Geometry: final body of the model. Coordinates: model frame, mm. Face numbers are marked on the shaded views. A direction names the side the tool comes from. Give positions to 0.01 mm unless a question says otherwise; leave off trailing zeros. Order: outer loops, then holes, each group sorted by start corner. A loop starts at its lowest first (then second) coordinate and runs counter-clockwise, first axis right, second up. Notation, with made-up numbers: M 25,-21.75 L 62,-21.75 A32 ccw 62,14.25 Z; hole C -34.5,0.25 d2. An arc over 180 degrees is marked long. Use CSV: the item, a comma, the result in double quotes.
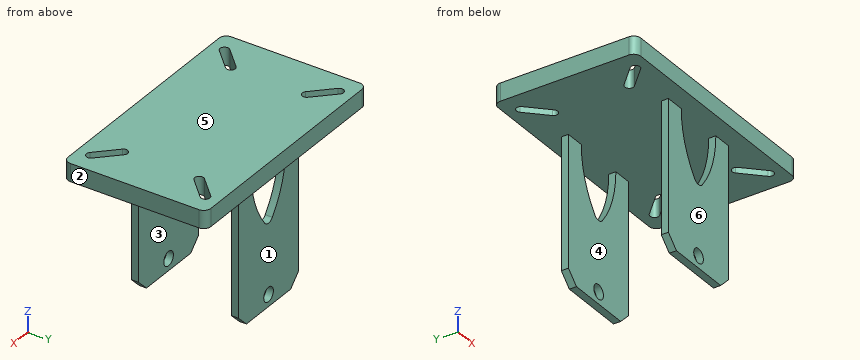
Autodesk Inventor part; units mm, degrees
ref_plane "Arbeitsebene1" through (0, 6, 0) normal (0, 1, 0) x (-1, 0, 0)
ref_plane "Arbeitsebene2" through (0, 6, 0) normal (0, 1, 0) x (-1, 0, 0)
ref_plane "YZ Plane" through (0, 0, 0) normal (1, 0, 0) x (0, 1, 0)
sketch "Skizze1" plane through (0, 0, 0) normal (0, 0, 1) x (1, 0, 0)
  line L0 (0, 0) -> (20, 0)
  line L1 (20, 0) -> (20, 12)
  line L2 (20, 12) -> (0, 12)
  line L3 (0, 12) -> (0, 0)
  point P0 (0, 6)
  dimension "d0" = 20
  dimension "d1" = 12
extrude "Extrusion1" add sketch "Skizze1" along normal blind 1.5
sketch "Skizze2" plane through (0, 0, 1.5) normal (0, 0, 1) x (1, 0, 0)
  line L0 (1.6868, 10.8132) -> (3.3132, 9.1868) construction
  line L1 (1.4217, 10.548) -> (3.048, 8.9217)
  line L2 (3.5783, 9.452) -> (1.952, 11.0783)
  arc A0 (1.952, 11.0783) -> (1.4217, 10.548) centre (1.6868, 10.8132) ccw
  arc A1 (3.048, 8.9217) -> (3.5783, 9.452) centre (3.3132, 9.1868) ccw
  line L3 (0, 12) -> (0, 0)
  line L4 (18.3132, 10.8132) -> (16.6868, 9.1868) construction
  line L5 (18.5783, 10.548) -> (16.952, 8.9217)
  line L6 (16.4217, 9.452) -> (18.048, 11.0783)
  arc A2 (18.5783, 10.548) -> (18.048, 11.0783) centre (18.3132, 10.8132) ccw
  arc A3 (16.4217, 9.452) -> (16.952, 8.9217) centre (16.6868, 9.1868) ccw
  line L7 (20, 0) -> (20, 12)
  line L8 (0, 0) -> (20, 0)
  line L9 (10, 0) -> (10, 12) construction
  line L10 (20, 12) -> (0, 12)
  point P0 (2.5, 10)
  point P1 (17.5, 10)
  dimension "d7" = 15
  dimension "d8" = 7.5
  dimension "d9" = 0.75
  dimension "d10" = 2
  dimension "d11" = 2.3
  dimension "d12" = 45
extrude "Extrusion2" cut sketch "Skizze2" against normal up to surface (1.5 mm away) contours A0 L2 A1 L1 | L5 A3 L6 A2
ref_plane "Arbeitsebene1" through (0, 6, 0) normal (0, 1, 0) x (-1, 0, 0)
mirror "Spiegeln1" about plane through (0, 6, 0) normal (0, 1, 0) of "Extrusion2"
sketch "Skizze3" plane through (0, 0, 0) normal (0, 0, -1) x (-1, 0, 0)
  line L0 (-20, 12) -> (0, 12)
  line L1 (-10, 12) -> (-10, 0) construction
  line L2 (0, 0) -> (-20, 0)
  line L3 (-6.25, 10.5) -> (-13.75, 10.5)
  line L4 (-13.75, 10.5) -> (-13.75, 9.9)
  line L5 (-13.75, 9.9) -> (-6.25, 9.9)
  line L6 (-6.25, 9.9) -> (-6.25, 10.5)
  dimension "d16" = 1.5
  dimension "d17" = 7.5
  dimension "d18" = 0.6
extrude "Extrusion3" add sketch "Skizze3" along normal blind 12
chamfer "Fasen1" distance 1 angle 45 2 edges at (13.75, 10.2, -12) (6.25, 10.2, -12)
sketch "Skizze4" plane through (6.25, 10.5, 0) normal (0, 1, 0) x (1, 0, 0)
  line L0 (7.5, 0) -> (0, 0)
  line L1 (3.75, 0) -> (3.75, 5.4569) construction
  arc A0 (5.9, 0) -> (3.75, 5.4569) centre (-2.1, 0) ccw
  arc A1 (3.75, 5.4569) -> (1.6, 0) centre (9.6, 0) ccw
  line L2 (13.75, 0) -> (-6.25, 0)
  line L3 (7.5, 0) -> (7.5, 11)
  dimension "d24" = 8
  dimension "d25" = 1.6
extrude "Extrusion4" cut sketch "Skizze4" against normal up to surface (0.6 mm away)
fillet "Rundung1" radius 0.6 1 edges at (10, 10.2, -5.4569)
sketch "Skizze5" plane through (7.25, 10.5, -12) normal (0, 1, 0) x (1, 0, 0)
  circle A0 centre (2.75, -1) radius 0.6
  line L0 (0, 0) -> (5.5, 0)
  line L1 (-1, -12) -> (-1, -1)
  point P0 (-7.25, -12)
  point P1 (2.75, 0)
  dimension "d30" = 1
  dimension "d31" = 1.2
extrude "Extrusion5" cut sketch "Skizze5" against normal up to surface (0.6 mm away)
ref_plane "Arbeitsebene2" through (0, 6, 0) normal (0, 1, 0) x (-1, 0, 0)
mirror "Spiegeln2" about plane through (0, 6, 0) normal (0, 1, 0) of "Extrusion3", "Extrusion4", "Extrusion5", "Fasen1", "Rundung1"
fillet "Rundung2" radius 0.6 4 edges at (20, 12, 0.75) (0, 12, 0.75) (0, 0, 0.75) (20, 0, 0.75)
properties part number "Koerper" material "Stahl, galvanisiert"
1. Reachability of the marked faces 1, 2 and 3 from +Z, -Z, +X, -X, +Y, -Y: full face, straight path, thin tool, end or side. Return the list, or none.
Answer:
face 1,"-Z, +X, -X, +Y"
face 2,"+Z, -Z, +X, +Y, -Y"
face 3,"-Z, +X, -X"
2. Section D-D, the plane y = 10.25. Give the number of separate pieces and of enclosed holes in the cut face, plus the area to 3 significant figures.
Answer:
separate pieces,"3"
enclosed holes,"2"
area,"98.7 mm2"
3. Pin query (flat end, axial travel): pin 1 Ø2 at (x, z) = (6.5, -10) entering from +Y; pin 2 Ø4 at (x, z) = (10.5, -6) entering from -Y; pin 3 Ø3 at (y, z) = (9, -3) entering from -X. Return the tip coordinate at first contact, or that it passes through.
Answer:
pin 1,"y = 10.5"
pin 2,"y = 1.5"
pin 3,"x = 6.25"
4. Line query: line 1 (Z direction, x = 10, y = 10.35); line 2 (Y direction, x = 8.5, z = -5.25); line 3 (Z direction, x = 19, y = 6.25). Output: solid intervals per line, ascending.
Answer:
line 1,"-12 to -11.6, -10.4 to -5.13, 0 to 1.5"
line 2,"1.5 to 2.1, 9.9 to 10.5"
line 3,"0 to 1.5"
5. Section B-B, the plane z = -7.5. Return the cut outline in (x, y).
Answer:
outline,"M 6.25,1.5 L 13.75,1.5 L 13.75,2.1 L 6.25,2.1 Z; M 6.25,9.9 L 13.75,9.9 L 13.75,10.5 L 6.25,10.5 Z"
6. Section A-A, the plane z = 0.75. Return the cut outline in (x, y).
Answer:
outline,"M 0,0.6 A0.6 ccw 0.6,0 L 19.4,0 A0.6 ccw 20,0.6 L 20,11.4 A0.6 ccw 19.4,12 L 0.6,12 A0.6 ccw 0,11.4 Z; hole M 1.42,1.45 A0.37 ccw 1.95,0.92 L 3.58,2.55 A0.37 ccw 3.05,3.08 Z; hole M 1.42,10.55 L 3.05,8.92 A0.37 ccw 3.58,9.45 L 1.95,11.08 A0.37 ccw Z; hole M 16.42,2.55 L 18.05,0.92 A0.37 ccw 18.58,1.45 L 16.95,3.08 A0.37 ccw Z; hole M 16.42,9.45 A0.37 ccw 16.95,8.92 L 18.58,10.55 A0.37 ccw 18.05,11.08 Z"
7. Pull-direction query (Y, two-part tool) for the marked faces 4, 5 and 6; classes: +Y half, -Y half, draft (parallel to the pull), parting line (faces both ways), or undercut.
Answer:
face 4,"undercut"
face 5,"draft"
face 6,"-Y half"
8. Section C-C, the plane x = 11.5. Return the cut outline in (y, z).
Answer:
outline,"M 0,0 L 12,0 L 12,1.5 L 0,1.5 Z; M 1.5,-12 L 2.1,-12 L 2.1,-3.16 L 1.5,-3.16 Z; M 9.9,-12 L 10.5,-12 L 10.5,-3.16 L 9.9,-3.16 Z"
